from build123d import *

# Parameters (mm, degrees)
SKETCH1_W           = 42.164
SKETCH1_H           = 42.164
BOSS_EXTRUDE1_DEPTH = 39.37
SKETCH1_3_W         = 16.0782
SKETCH1_3_H         = 6.096
BOSS_EXTRUDE2_DEPTH = 9.144
SKETCH2_R           = 10.9855
BOSS_EXTRUDE3_DEPTH = 2.286
SKETCH3_R           = 2.54
BOSS_EXTRUDE4_DEPTH = 21.844
SKETCH4_R           = 1.27
CUT_EXTRUDE1_DEPTH  = 6.35
CUT_EXTRUDE2_DEPTH  = 40.37
FILLET1_R           = 1.27


with BuildPart() as part:
    # Sketch1 → Boss-Extrude1 (new body)
    with BuildSketch(Plane(origin=(0, 0, 0), x_dir=(1, 0, 0), z_dir=(0, 1, 0))):
        Rectangle(SKETCH1_W, SKETCH1_H)
    extrude(amount=BOSS_EXTRUDE1_DEPTH)

    # Sketch1_3 → Boss-Extrude2 (add)
    with BuildSketch(Plane(origin=(0, 0, 0), x_dir=(1, 0, 0), z_dir=(0, 1, 0))):
        with Locations((0, -24.13)):
            Rectangle(SKETCH1_3_W, SKETCH1_3_H)
    extrude(amount=BOSS_EXTRUDE2_DEPTH)

    # Sketch2 → Boss-Extrude3 (add)
    with BuildSketch(Plane(origin=(0, 39.37, 0), x_dir=(1, 0, 0), z_dir=(0, 1, 0))):
        Circle(SKETCH2_R)
    extrude(amount=BOSS_EXTRUDE3_DEPTH)

    # Sketch3 → Boss-Extrude4 (add)
    with BuildSketch(Plane(origin=(0, 41.656, 0), x_dir=(1, 0, 0), z_dir=(0, 1, 0))):
        Circle(SKETCH3_R)
    extrude(amount=BOSS_EXTRUDE4_DEPTH)

    # Sketch4 → Cut-Extrude1 (cut)
    with BuildSketch(Plane(origin=(0, 39.37, 0), x_dir=(1, 0, 0), z_dir=(0, 1, 0))):
        with Locations((-15.494, 15.494)):
            Circle(SKETCH4_R)
        with Locations((15.494, 15.494)):
            Circle(SKETCH4_R)
        with Locations((15.494, -15.494)):
            Circle(SKETCH4_R)
        with Locations((-15.494, -15.494)):
            Circle(SKETCH4_R)
    extrude(amount=-CUT_EXTRUDE1_DEPTH, mode=Mode.SUBTRACT)

    # Sketch5 → Cut-Extrude2 (cut, through all)
    with BuildSketch(Plane(origin=(0, 39.37, 0), x_dir=(1, 0, 0), z_dir=(0, 1, 0))):
        Polygon((-21.082, 16.51), (-16.51, 21.082), (-21.082, 21.082), align=None)
        Polygon((16.51, 21.082), (21.082, 16.51), (21.082, 21.082), align=None)
        Polygon((21.082, -16.51), (16.51, -21.082), (21.082, -21.082), align=None)
        Polygon((-16.51, -21.082), (-21.082, -16.51), (-21.082, -21.082), align=None)
    extrude(amount=-CUT_EXTRUDE2_DEPTH, mode=Mode.SUBTRACT)

    # Fillet1
    fillet1_edges = [part.edges().sort_by_distance(p)[0] for p in [
        (-16.51, 19.685, 21.082),
        (-21.082, 19.685, 16.51),
        (21.082, 19.685, 16.51),
        (16.51, 19.685, 21.082),
        (16.51, 19.685, -21.082),
        (21.082, 19.685, -16.51),
        (-21.082, 19.685, -16.51),
        (-16.51, 19.685, -21.082),
    ]]
    fillet(fillet1_edges, radius=FILLET1_R)


solid = part.part
Can you work these out from the model? Positions are in its coordinate system, mm. A direction names the side the tool comes from. Give positions to 0.01 mm unless a question says otherwise; leave off trailing zeros. Loops run counter-clockwise (first coordinate to the right, second up) from the corner with the lowest first, then second, coordinate; pieces in that order, holes last. Notation, with made-up numbers: M -32,45.5 L 15,45.5 A29 ccw 15,68.5 Z; hole C -0.5,46.25 d8. An arc over 180 degrees is marked long. One line per item, written item: value.
1) On a 3-axis mill with a long thin cutter (end or side, diameter ignored), from which of +Z, -Z, +X, -X, +Y, -Y can I reach the whole of each face in a straight line? I mean faces 4 (the face through (0, 9.144, 24)), 5 (the face through (15, 33.02, -16)), 6 (the face through (8.039, 5, 24)). Say none if no direction works.
Geometry check:
face 4: +Z, +X, -X, +Y
face 5: +Y
face 6: +Z, +X, +Y, -Y
2) Imagine slicing it at A-A on x = 0. Write out the boundary of the cut face in (y, z).
Geometry check:
outline: M 0,-21.08 L 39.37,-21.08 L 39.37,-10.99 L 41.66,-10.99 L 41.66,-2.54 L 63.5,-2.54 L 63.5,2.54 L 41.66,2.54 L 41.66,10.99 L 39.37,10.99 L 39.37,21.08 L 9.14,21.08 L 9.14,27.18 L 0,27.18 Z
3) Imagine slicing it at C-C on z = -7.5. Write out the boundary of the cut face in (x, y).
Geometry check:
outline: M -21.08,0 L 21.08,0 L 21.08,39.37 L 8.03,39.37 L 8.03,41.66 L -8.03,41.66 L -8.03,39.37 L -21.08,39.37 Z
4) I'm going to push flat-ended pins straight in: pin 1 (9.5 mm diameter, centred on x = 4, y = 17.5, fed in from +Z); pin 2 (0.8 mm diameter, centred on x = -15, z = 15.5, fed in from +Y); pin 3 (1.8 mm diameter, centred on y = 4.5, z = 24.5, fed in from -X). Where does each tip first touch, or does it pass through?
Geometry check:
pin 1: stops at z = 21.08
pin 2: stops at y = 33.02
pin 3: stops at x = -8.04
5) Imagine slicing it at B-B on y = 31.5. Write out the boundary of the cut face in (x, z).
Geometry check:
outline: M -21.08,-15.98 A1.27 ccw -20.71,-16.88 L -16.88,-20.71 A1.27 ccw -15.98,-21.08 L 15.98,-21.08 A1.27 ccw 16.88,-20.71 L 20.71,-16.88 A1.27 ccw 21.08,-15.98 L 21.08,15.98 A1.27 ccw 20.71,16.88 L 16.88,20.71 A1.27 ccw 15.98,21.08 L -15.98,21.08 A1.27 ccw -16.88,20.71 L -20.71,16.88 A1.27 ccw -21.08,15.98 Z
6) Thinking about a two-plate mould opening in Z: for faces 1 (the face through (0, 0, 3)), 2 (the face through (15.219, 36.239, 16.734)), 3 (the face through (18.82, 19.96, 18.77)), which applies, +Z half, -Z half, draft (parallel to the pull), parting line (faces both ways), or undercut?
Geometry check:
face 1: draft
face 2: undercut
face 3: +Z half
7) Imagine slicing it at D-D on y = 4.5. Write out the boundary of the cut face in (x, z), and give its area (3 significant figures).
Geometry check:
outline: M -21.08,-15.98 A1.27 ccw -20.71,-16.88 L -16.88,-20.71 A1.27 ccw -15.98,-21.08 L 15.98,-21.08 A1.27 ccw 16.88,-20.71 L 20.71,-16.88 A1.27 ccw 21.08,-15.98 L 21.08,15.98 A1.27 ccw 20.71,16.88 L 16.88,20.71 A1.27 ccw 15.98,21.08 L 8.04,21.08 L 8.04,27.18 L -8.04,27.18 L -8.04,21.08 L -15.98,21.08 A1.27 ccw -16.88,20.71 L -20.71,16.88 A1.27 ccw -21.08,15.98 Z
area: 1,830 mm²
8) Please list where these lines run through material, in increasing order: line 1 (Y direction, x = 0.5, z = 17); line 2 (Y direction, x = -7, z = 23); line 3 (Z direction, x = 1, y = 23.5).
Geometry check:
line 1: y = 0 to 39.37
line 2: y = 0 to 9.14
line 3: z = -21.08 to 21.08
